from build123d import *

# Parameters (mm, degrees)
THICKEN1_T1 = 2


with BuildPart() as body_1:
    # Sketch6 → Surface-Plane1: a flat surface bounded by the sketch
    with BuildSketch(Plane(origin=(220, 0, 0), x_dir=(0, 0, -1), z_dir=(1, 0, 0)), mode=Mode.PRIVATE) as surface_plane1_1_region:
        with BuildLine():
            Line((10.544114441, 47.367154835), (109.327040639, 47.367154835))
            ThreePointArc((109.327040639, 47.367154835), (118.816017042, 44.972816618), (126.033011561, 38.363087517))
            Line((126.033011561, 38.363087517), (151.900895956, -0.937637305))
            ThreePointArc((151.900895956, -0.937637305), (152.800586817, -21.422546391), (135.194925034, -31.933569988))
            Line((135.194925034, -31.933569988), (-15.358621791, -31.933569988))
            ThreePointArc((-15.358621791, -31.933569988), (-32.967217144, -21.417101487), (-32.05778866, -0.927306957))
            Line((-32.05778866, -0.927306957), (-6.155052428, 38.373417866))
            ThreePointArc((-6.155052428, 38.373417866), (1.060582941, 44.975750188), (10.544114441, 47.367154835))
        make_face()
    surface_plane1_1 = surface_plane1_1_region.sketch.faces()[0]
    add(Solid.thicken(surface_plane1_1, THICKEN1_T1))


solid = body_1.part
Can you work these out from the model? Positions are in its coordinate system, mm. Give positions to 0.01 mm unless a question says otherwise; leave off trailing zeros. Loops run counter-clockwise (first coordinate to the right, second up) from the corner with the lowest first, then second, coordinate; pieces in that order, holes last. Notation, with made-up numbers: (-18, 65.5) -> (1, 65.5) arc R10 cw to (1, 79.5) -> close; hole circle Ø6 at (6, 68). An arc over 180 degrees is marked (long way). Return JSON: item names as keys, results as strings.
Q1. I want a section at A-A, the plane x = 220.8. List the corners of the cut face in (y, z) for me, then the cut area to 3 significant figures.
Checks:
{"outline": "(-31.93, -135.19) arc R20 ccw to (-0.94, -151.9) -> (38.36, -126.03) arc R20 ccw to (47.37, -109.33) -> (47.37, -10.54) arc R20 ccw to (38.37, 6.16) -> (-0.93, 32.06) arc R20 ccw to (-31.93, 15.36) -> close", "area": "13,000 mm2"}
Q2. I want a section at B-B, the plane z = 20.5. List the corners of the cut face in (x, y) for me, then the cut area to 3 significant figures.
Checks:
{"outline": "(220, -31.26) -> (222, -31.26) -> (222, 16.61) -> (220, 16.61) -> close", "area": "95.7 mm2"}
Q3. I need wall thicknesses on probe 1 along Z at (x, y) = (221.6, -12); probe 2 along Z at (x, y) = (221.65, -23.5); probe 3 along Y at (x, z) = (221.4, 12.5). Which ranges of each line are inside material? Lowest first, please.
Checks:
{"probe 1": "z = -155.19 to 35.36", "probe 2": "z = -151.51 to 31.67", "probe 3": "y = -31.93 to 28.75"}
Q4. I want a section at C-C, the plane y = 21.5. List the corners of the cut face in (x, z) for me, then the cut area to 3 significant figures.
Checks:
{"outline": "(220, -137.13) -> (222, -137.13) -> (222, 17.28) -> (220, 17.28) -> close", "area": "309 mm2"}
